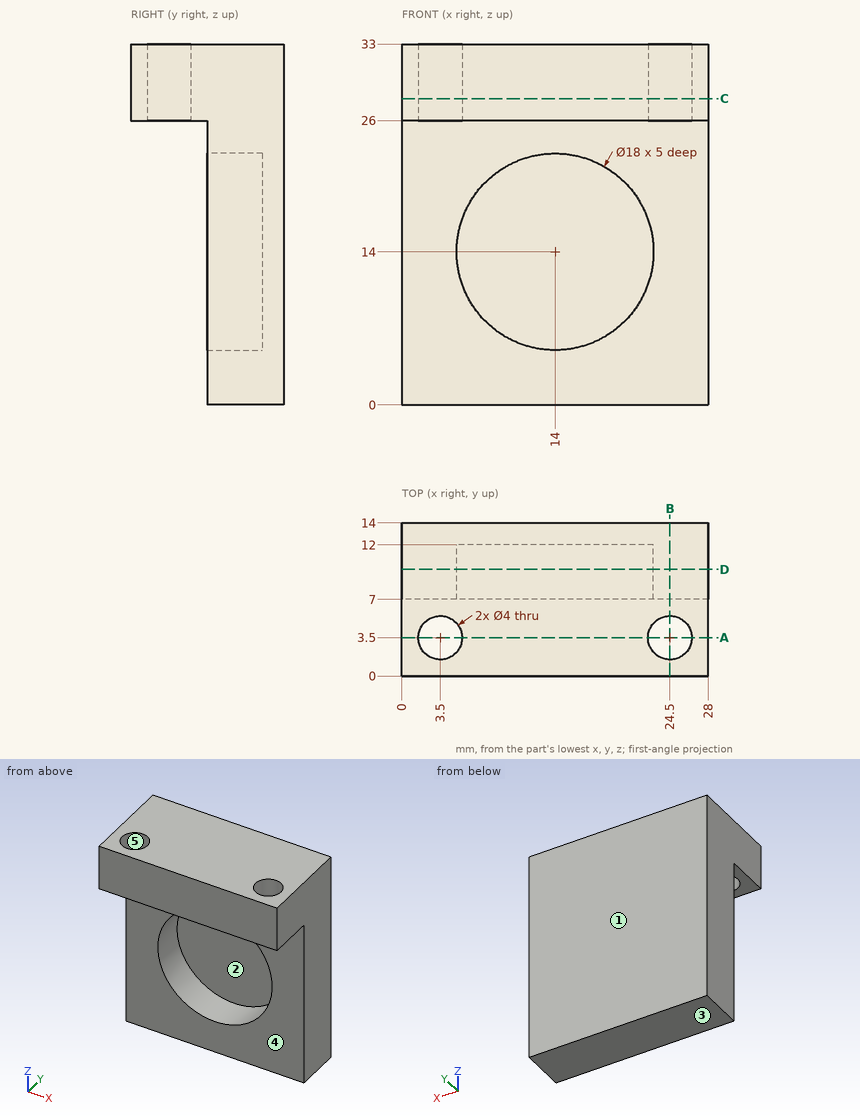
Input: dimensioned drawing with shaded views. Units: mm. Origin: part minimum x, y, z. A direction names the side the tool comes from. Coordinates: 2 decimals unless noted, no trailing zeros. Loops run counter-clockwise (first coordinate to the right, second up) from the corner with the lowest first, then second, coordinate; pieces in that order, holes last. Notation, with made-up numbers: (36.25, 6) -> (48.25, 6) arc R33 cw to (48.25, 34) -> close; hole circle Ø8 at (36.25, 14.25). An arc over 180 degrees is marked (long way). Use a Markdown table: item, result. Add a question column.
(1) Section query A-A, the plane y = 3.5. Return loops of the section in (x, z), plus the area to 3 significant figures.
(2) Section query D-D, the plane y = 9.75. Return loops of the section in (x, z).
(3) Section query C-C, the plane z = 28. Return loops of the section in (x, y), plus the area to 3 significant figures.
(4) Line query: line 1 along Y through (x, z) = (24.5, 32); line 2 along X through (y, z) = (9.5, 14); line 3 along Y through (x, z) = (13.5, 2.5). Output: solid intervals per line, ascending.
(5) Mould query, pull axis Y, two halves, no side actions, for the marked faces 3, 4 and 5. Classes: pulls with the +Y half, pulls with the -Y half, needs draft (parallel to the pull), parting line crosses it, or undercut.
(6) Pin query (flat end, axial travel): pin 1 Ø2 at (x, y) = (14.5, 4) entering from -Z; pin 2 Ø2 at (x, z) = (9, 10.5) entering from -Y; pin 3 Ø1 at (x, z) = (3, 3.5) entering from -Y. Return the tip coordinate at first contact, or that it passes through.
(7) Section query B-B, the plane x = 24.5. Return loops of the section in (y, z), plus the area to 3 significant figures.
(8) Access query for the marked faces 1 and 2. Directions: +Z, -Z, +X, -X, +Y, -Y. A direction counts if a zero-diameter tool reaches every point of the face in a straight line with its end or side. Return the directions, or none.
Answer:
| question | item | result |
|---|---|---|
| 1 | outline | (0, 26) -> (1.5, 26) -> (1.5, 33) -> (0, 33) -> close; (5.5, 26) -> (22.5, 26) -> (22.5, 33) -> (5.5, 33) -> close; (26.5, 26) -> (28, 26) -> (28, 33) -> (26.5, 33) -> close |
| 1 | area | 140 mm^2 |
| 2 | outline | (0, 0) -> (28, 0) -> (28, 33) -> (0, 33) -> close; hole circle Ø18 at (14, 14) |
| 3 | outline | (0, 0) -> (28, 0) -> (28, 14) -> (0, 14) -> close; hole circle Ø4 at (3.5, 3.5); hole circle Ø4 at (24.5, 3.5) |
| 3 | area | 367 mm^2 |
| 4 | line 1 | y = 0 to 1.5, 5.5 to 14 |
| 4 | line 2 | x = 0 to 5, 23 to 28 |
| 4 | line 3 | y = 7 to 14 |
| 5 | face 3 | needs draft |
| 5 | face 4 | pulls with the -Y half |
| 5 | face 5 | undercut |
| 6 | pin 1 | stops at z = 26 |
| 6 | pin 2 | stops at y = 12 |
| 6 | pin 3 | stops at y = 7 |
| 7 | outline | (0, 26) -> (1.5, 26) -> (1.5, 33) -> (0, 33) -> close; (5.5, 26) -> (7, 26) -> (7, 0) -> (14, 0) -> (14, 33) -> (5.5, 33) -> close |
| 7 | area | 252 mm^2 |
| 8 | face 1 | +Z, -Z, +X, -X, +Y |
| 8 | face 2 | -Y |
